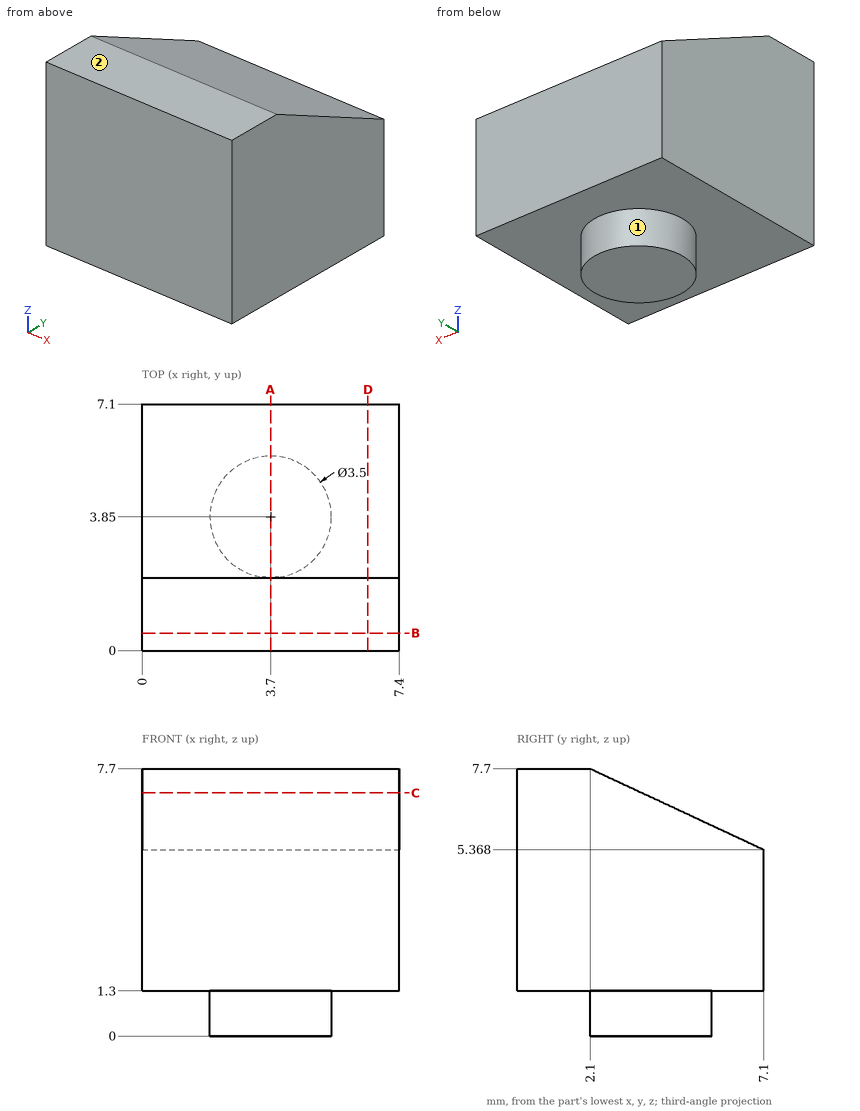
Geometry: see drawing. Coordinates: mm, zero at the bounding-box minimum. A direction names the side the tool comes from. Give positions to 0.01 mm unless a question says otherwise; leave off trailing zeros. Order: outer loops, then holes, each group sorted by start corner. A loop starts at its lowest first (then second) coordinate and runs counter-clockwise, first axis right, second up. Notation, with made-up numbers: M 62.5,23.5 L 115.5,23.5 A23 ccw 115.5,52.5 Z; hole C 70.25,40 d2. An arc over 180 degrees is marked long. Answer as a JSON object with one key per item and string values.
1. First-contact query: P1, Ø1.5, axis at x = 4, y = 4.5, coming from the +Z side; P2, Ø2, axis at x = 5.5, y = 6.5, coming from the +Z side (1 decimal); P3, Ø4, axis at x = 4, y = 6, coming from the +Z side (1 decimal). Flat tips, straight axial feed; report the tip coordinate or a pass-through.
Result sheet:
{"P1": "z = 6.93", "P2": "z = 6.1", "P3": "z = 6.8"}
2. Cut plane B-B, the plane y = 0.5. Output: boundary loops of the cut face in (x, z).
Result sheet:
{"outline": "M 0,1.3 L 7.4,1.3 L 7.4,7.7 L 0,7.7 Z"}
3. Cut plane C-C, the plane z = 7. Output: boundary loops of the cut face in (x, y).
Result sheet:
{"outline": "M 0,0 L 7.4,0 L 7.4,3.6 L 0,3.6 Z"}
4. Ray query, line 1 (Z direction, x = 2.5, y = 1.5); line 2 (Y direction, x = 5, z = 7) (1 decimal); line 3 (Y direction, x = 7, z = 5.5) (1 decimal). Return the intervals inside material, ascending. Write a range as [from, to].
Result sheet:
{"line 1": "[1.3, 7.7]", "line 2": "[0, 3.6]", "line 3": "[0, 6.8]"}
5. Cut plane A-A, the plane x = 3.7. Output: boundary loops of the cut face in (y, z).
Result sheet:
{"outline": "M 0,1.3 L 2.1,1.3 L 2.1,0 L 5.6,0 L 5.6,1.3 L 7.1,1.3 L 7.1,5.37 L 2.1,7.7 L 0,7.7 Z"}
6. Reachability of the marked faces 1 and 2 from +Z, -Z, +X, -X, +Y, -Y: full face, straight path, thin tool, end or side. Return the list, or none.
Result sheet:
{"face 1": "-Z", "face 2": "+Z, +X, -X, +Y, -Y"}
7. Cut plane D-D, the plane x = 6.5. Output: boundary loops of the cut face in (y, z), and give its area (3 significant figures).
Result sheet:
{"outline": "M 0,1.3 L 7.1,1.3 L 7.1,5.37 L 2.1,7.7 L 0,7.7 Z", "area": "39.6 mm²"}
